from build123d import *

# Parameters (mm, degrees)
ESQUISSE1_R             = 11.5
BOSS_EXTRU_1_DEPTH      = 2
ESQUISSE6_RX            = 6
ESQUISSE6_RY            = 2.5
BOSS_EXTRU_5_DEPTH      = 2
ESQUISSE7_R             = 0.75
ENL_V_MAT_EXTRU_1_DEPTH = 17.748134224


with BuildPart() as part:
    # Esquisse1 → Boss.-Extru.1 (new body)
    with BuildSketch(Plane.XY):
        Circle(ESQUISSE1_R)
    extrude(amount=BOSS_EXTRU_1_DEPTH)

    # Esquisse6 → Boss.-Extru.5 (add)
    with BuildSketch(Plane.XY.offset(2)):
        with Locations((0, 0)):
            Ellipse(ESQUISSE6_RX, ESQUISSE6_RY)
    extrude(amount=BOSS_EXTRU_5_DEPTH)

    # Esquisse7 → Enlèv. mat.-Extru.1 (cut, through all)
    with BuildSketch(Plane(origin=(0, 0, 0), x_dir=(-1, 0, 0), z_dir=(0, 0, -1))):
        with Locations((1.650464666, 0)):
            Circle(ESQUISSE7_R)
        with Locations((-1.650464666, 0)):
            Circle(ESQUISSE7_R)
    extrude(amount=-ENL_V_MAT_EXTRU_1_DEPTH, mode=Mode.SUBTRACT)


solid = part.part
Here's how the part is built. I have some questions about the finished solid (model axes, mm). Round coordinates to 2 decimals unless told otherwise and drop trailing zeros. Order: outer loops, then holes, each group sorted by start corner. A loop starts at its lowest first (then second) coordinate and runs counter-clockwise, first axis right, second up. Notation, with made-up numbers: (38, -31) -> (64, -31) arc R20 cw to (64, -20) -> close; hole circle Ø8 at (42.5, -23.5). An arc over 180 degrees is marked (long way). Return JSON: item names as keys, results as strings.
Q1. If we section it at A-A on y = 0: Give the number of separate pieces and of enclosed holes in the cut face, plus the area to 3 significant figures.
Filled sheet:
{"separate pieces": "3", "enclosed holes": "0", "area": "58.0 mm^2"}
Q2. If we section it at C-C on x = 10.25: List the corners of the cut face in (y, z) for me, plus the area to 3 significant figures.
Filled sheet:
{"outline": "(-5.21, 0) -> (5.21, 0) -> (5.21, 2) -> (-5.21, 2) -> close", "area": "20.9 mm^2"}
Q3. I need wall thicknesses on line 1 along Z through (x, y) = (6, -6); line 2 along Y through (x, z) = (5.5, 0.95); line 3 along X through (y, z) = (4, 1.5). Which ranges of each line are inside material? Lowest first, please. Write a range as from..to.
Filled sheet:
{"line 1": "z = 0..2", "line 2": "y = -10.1..10.1", "line 3": "x = -10.78..10.78"}
Q4. If we section it at D-D on y = -3.75: List the corners of the cut face in (x, z) for me, plus the area to 3 significant figures.
Filled sheet:
{"outline": "(-10.87, 0) -> (10.87, 0) -> (10.87, 2) -> (-10.87, 2) -> close", "area": "43.5 mm^2"}
Q5. If we mould it in two halves opening along X, with no side actions, what happens to faces 1 (the flat face through (0, 0, 4)), 2 (the cylindrical face through (-2.366, 0.225, 1.972)), 3 (the cylindrical face through (-1.5, 11.4, 1))? For each: released by +X, released by -X, zero draft, split by the parting line, or undercut.
Filled sheet:
{"face 1": "zero draft", "face 2": "undercut", "face 3": "split by the parting line"}
Q6. For pin 1 Ø5 at (x, y) = (7, 4) entering from +Z, with a flat end and sliding along its axis, tell me the tip position at first contact or that it passes through.
Filled sheet:
{"pin 1": "stops at z = 2"}
